from build123d import *

# Parameters (mm, degrees)
BOSS_EXTRUDE1_DEPTH = 18.5
SKETCH2_W           = 15
SKETCH2_H           = 48
CUT_EXTRUDE1_DEPTH  = 15
SKETCH3_R           = 1.75
CUT_EXTRUDE2_DEPTH  = 3.5
SKETCH4_R           = 1.75
CUT_EXTRUDE3_DEPTH  = 4
SKETCH5_R           = 1.75
CUT_EXTRUDE4_DEPTH  = 4
CUT_EXTRUDE5_DEPTH  = 19
FILLET1_R           = 2
FILLET2_R           = 5
FILLET3_R           = 1


with BuildPart() as part:
    # Sketch1 → Boss-Extrude1 (new body)
    with BuildSketch(Plane.XY):
        Polygon((24.259932708, 13.808119809), (39.856078127, -34.191880191), (7.453399362, -34.191880191), (-14.546600638, -34.191880191), (-14.546600638, 13.808119809), align=None)
    extrude(amount=BOSS_EXTRUDE1_DEPTH)

    # Sketch2 → Cut-Extrude1 (cut)
    with BuildSketch(Plane.XY.offset(18.5)):
        with Locations((-3.546600638, -10.191880191)):
            Rectangle(SKETCH2_W, SKETCH2_H)
        Polygon((36.175960342, -34.191880191), (22.309194948, 8.485635376), (8.043347203, 3.85038046), (20.404026978, -34.191880191), align=None)
    extrude(amount=-CUT_EXTRUDE1_DEPTH, mode=Mode.SUBTRACT)

    # Sketch3 → Cut-Extrude2 (cut)
    with BuildSketch(Plane(origin=(26.001419868, 8.448373445, 0), x_dir=(0, 0, -1), z_dir=(0.9510565162951533, 0.3090169943749487, 0))):
        with Locations(Location((-11, -31.197396994, 0), (0, 0, 90))):
            Circle(SKETCH3_R)
        with Locations(Location((-11, -11.323601551, 0), (0, 0, 90))):
            Circle(SKETCH3_R)
    extrude(amount=-CUT_EXTRUDE2_DEPTH, mode=Mode.SUBTRACT)

    # Sketch4 → Cut-Extrude3 (cut)
    with BuildSketch(Plane(origin=(0, 0, 0), x_dir=(-1, 0, 0), z_dir=(0, 0, -1))):
        with Locations((-24.427281231, -22.303673738)):
            Circle(SKETCH4_R)
        with Locations((-19.038983505, -5.720198536)):
            Circle(SKETCH4_R)
        with Locations((3.546600638, 1.308119809)):
            Circle(SKETCH4_R)
        with Locations((3.546600638, -21.691880191)):
            Circle(SKETCH4_R)
    extrude(amount=-CUT_EXTRUDE3_DEPTH, mode=Mode.SUBTRACT)

    # Sketch5 → Cut-Extrude4 (cut)
    with BuildSketch(Plane.ZY.offset(14.546600638)):
        with Locations(Location((11, -21.691880191, 0), (0, 0, 270))):
            Circle(SKETCH5_R)
        with Locations(Location((11, 1.308119809, 0), (0, 0, 270))):
            Circle(SKETCH5_R)
    extrude(amount=-CUT_EXTRUDE4_DEPTH, mode=Mode.SUBTRACT)

    # Sketch6 → Cut-Extrude5 (cut)
    with BuildSketch(Plane.XY.offset(18.5)):
        Polygon((36.175960342, -34.191880191), (39.504658149, -33.110320711), (39.856078127, -34.191880191), align=None)
    extrude(amount=-CUT_EXTRUDE5_DEPTH, mode=Mode.SUBTRACT)

    # Fillet1
    fillet1_edges = [part.edges().sort_by_distance(p)[0] for p in [
        (39.504658149, -33.110320711, 9.25),
    ]]
    fillet(fillet1_edges, radius=FILLET1_R)

    # Fillet2
    fillet2_edges = [part.edges().sort_by_distance(p)[0] for p in [
        (24.259932708, 13.808119809, 9.25),
    ]]
    fillet(fillet2_edges, radius=FILLET2_R)

    # Fillet3
    fillet3_edges = [part.edges().sort_by_distance(p)[0] for p in [
        (36.889252729, -33.960117446, 18.5),
        (38.766524176, -32.734222667, 18.5),
        (32.134563405, -10.427501449, 18.5),
        (23.566146329, 12.85320478, 18.5),
        (36.889252729, -33.960117446, 0),
        (38.766524176, -32.734222667, 0),
        (32.134563405, -10.427501449, 0),
        (23.566146329, 12.85320478, 0),
        (12.17871317, -34.191880191, 18.5),
        (12.290309715, 13.808119809, 18.5),
        (-14.546600638, -34.191880191, 9.25),
        (-14.546600638, 13.808119809, 9.25),
        (-14.546600638, -10.191880191, 18.5),
        (10.814679852, -34.191880191, 0),
        (3.040309715, 13.808119809, 0),
        (-14.546600638, -10.191880191, 0),
    ]]
    fillet(fillet3_edges, radius=FILLET3_R)


solid = part.part
Here's how the part is built. I have some questions about the finished solid (model axes, mm). A direction names the side the tool comes from. Give positions to 0.01 mm unless a question says otherwise; leave off trailing zeros. Order: outer loops, then holes, each group sorted by start corner. A loop starts at its lowest first (then second) coordinate and runs counter-clockwise, first axis right, second up. Notation, with made-up numbers: (-18, -40) -> (15, -40) arc R26 ccw to (15, -20) -> close; hole circle Ø6 at (23, 80). An arc over 180 degrees is marked (long way). Use a Markdown table: item, result. Add a question column.
Item 1: Imagine slicing it at A-A on z = 16.25. Please give me the cut outline in (x, y), plus the area to 3 significant figures.
Item 2: If we mould it in two halves opening along X, with no side actions, what happens to faces 5 (the face through (33.71, -20.861, 12.476)), 6 (the face through (14, -15, 18.5)), 7 (the face through (14.137, -14.904, 11.105)), 8 (the face through (36.879, -33.963, 9.366))? For each: pulls with the +X half, pulls with the -X half, needs draft (parallel to the pull), parting line crosses it, or undercut.
Item 3: Imagine slicing it at B-B on z = 11. Give the number of separate pieces and of enclosed holes in the cut face, plus the area to 3 significant figures.
Item 4: Will these pins go through, and if not, where does the flat tip stop? pin 1 (10 mm diameter, centred on x = 19, y = 1.5, fed in from +Z); pin 2 (5.5 mm diameter, centred on y = 1.31, z = 11, fed in from +X); pin 3 (5 mm diameter, centred on y = -25, z = 5.5, fed in from +X).
Item 5: I need wall thicknesses on line 1 (X direction, y = -22, z = 15.5); line 2 (X direction, y = -17.5, z = 5.75); line 3 (Z direction, x = 13, y = 2). Which ranges of each line are inside material? Lowest first, please.
Item 6: For faces 1 (the face through (29.34, -13.15, 11.1)), 2 (the face through (-11.047, -11, 11)), 3 (the face through (-12.82, -23.36, 11.53)), 4 (the face through (15.28, 6.2, 11.1)), which set-ups out of +Z, -Z, +X, -X, +Y, -Y let a thin tool reach every point of the face, with its end or its side?
Item 7: Imagine slicing it at C-C on x = 2.5. Please give me the cut outline in (y, z).
Data:
| question | item | result |
|---|---|---|
| 1 | outline | (-14.55, -33.19) arc R1 ccw to (-13.55, -34.19) -> (-11.05, -34.19) -> (-11.05, 13.81) -> (-13.55, 13.81) arc R1 ccw to (-14.55, 12.81) -> close; (3.95, -34.19) -> (20.4, -34.19) -> (8.04, 3.85) -> (22.31, 8.49) -> (36.18, -34.19) -> (37.6, -33.73) arc R2 ccw to (38.89, -31.21) -> (25.38, 10.35) arc R5 ccw to (20.63, 13.81) -> (3.95, 13.81) -> close |
| 1 | area | 875 mm² |
| 2 | face 5 | undercut |
| 2 | face 6 | needs draft |
| 2 | face 7 | undercut |
| 2 | face 8 | pulls with the +X half |
| 3 | separate pieces | 6 |
| 3 | enclosed holes | 0 |
| 3 | area | 826 mm² |
| 4 | pin 1 | stops at z = 3.5 |
| 4 | pin 2 | stops at x = 29.12 |
| 4 | pin 3 | stops at x = 37.68 |
| 5 | line 1 | x = -14.55 to -11.05, 3.95 to 16.44, 32.21 to 35.89 |
| 5 | line 2 | x = -14.55 to -11.05, 3.95 to 14.98, 30.75 to 34.43 |
| 5 | line 3 | z = 0 to 3.5 |
| 6 | face 1 | +Z, -Y |
| 6 | face 2 | +Z, +Y, -Y |
| 6 | face 3 | -X |
| 6 | face 4 | +Z |
| 7 | outline | (-34.19, 1) arc R1 ccw to (-33.19, 0) -> (12.81, 0) arc R1 ccw to (13.81, 1) -> (13.81, 3.5) -> (-34.19, 3.5) -> close |
